Read the model definition and answer for the solid it produces. Units are mm, in the model's axes. Coordinates: 2 decimals unless noted, no trailing zeros. Loops run counter-clockwise (first coordinate to the right, second up) from the corner with the lowest first, then second, coordinate; pieces in that order, holes last. Notation, with made-up numbers: M 68,67.25 L 99,67.25 A22 cw 99,83.25 Z; hole C 41.5,55 d11. An arc over 180 degrees is marked long. Use one line per item in the form item = value. Start each with the question number.
1. Find the intervals of material crossed by probe 1 along Y at (x, z) = (0, 1.5); probe 2 along Z at (x, y) = (-20.5, 0); probe 3 along X at (y, z) = (6, 3), in increasing order. Write a range as [from, to].
2. The part is cut by section B-B (x = 80.5). Give the vertices of the cut face in (y, z), plus the area to 3 significant figures.
3. Flat-ended cylindrical pins translate along their axes: pin 1 (2.5 mm diameter, centred on x = -7.07, y = 7.07, fed in from +Z) (3 decimals); pin 2 (2 mm diameter, centred on x = 46, z = -2, fed in from +Y). Find the tip coordinate at first contact, or state that the pin passes through.
4. The part is cut by section A-A (z = 0). Give the number of separate pieces and of enclosed holes in the cut face, plus the area to 3 significant figures.
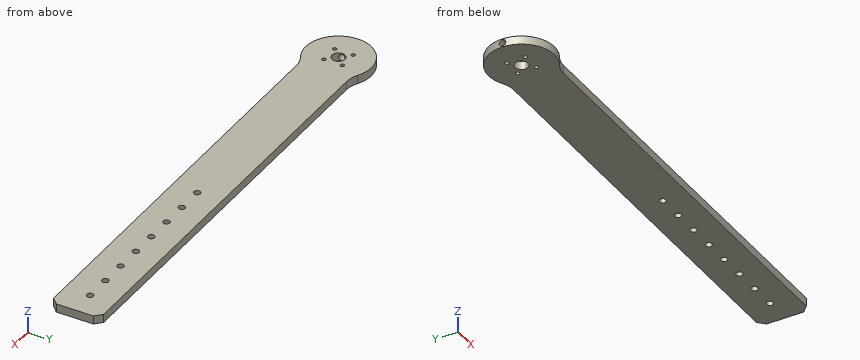
from build123d import *

# Parameters (mm, degrees)
SKETCH1_R           = 1.5
SKETCH1_R_2         = 2.5
SKETCH1_R_3         = 5
BOSS_EXTRUDE1_DEPTH = 3.2
SKETCH4_R           = 2.5
CUT_EXTRUDE1_DEPTH  = 32.4
FILLET1_R           = 20
CHAMFER1_SIZE       = 5


with BuildPart() as part:
    # Sketch1 → Boss-Extrude1 (new, symmetric)
    with BuildSketch(Plane.XY):
        with BuildLine():
            Line((345, 19.05), (16.189425561, 19.05))
            ThreePointArc((16.189425561, 19.05), (-25, 0), (16.189425561, -19.05))
            Line((16.189425561, -19.05), (345, -19.05))
            Line((345, -19.05), (345, 19.05))
        make_face()
        with Locations((7.071067812, 7.071067812)):
            Circle(SKETCH1_R, mode=Mode.SUBTRACT)
        with Locations((7.071067812, -7.071067812)):
            Circle(SKETCH1_R, mode=Mode.SUBTRACT)
        with Locations((-7.071067812, -7.071067812)):
            Circle(SKETCH1_R, mode=Mode.SUBTRACT)
        with Locations((-7.071067812, 7.071067812)):
            Circle(SKETCH1_R, mode=Mode.SUBTRACT)
        with Locations((325, 0)):
            Circle(SKETCH1_R_2, mode=Mode.SUBTRACT)
        with Locations((305, 0)):
            Circle(SKETCH1_R_2, mode=Mode.SUBTRACT)
        with Locations((285, 0)):
            Circle(SKETCH1_R_2, mode=Mode.SUBTRACT)
        with Locations((265, 0)):
            Circle(SKETCH1_R_2, mode=Mode.SUBTRACT)
        with Locations((245, 0)):
            Circle(SKETCH1_R_2, mode=Mode.SUBTRACT)
        with Locations((225, 0)):
            Circle(SKETCH1_R_2, mode=Mode.SUBTRACT)
        with Locations((205, 0)):
            Circle(SKETCH1_R_2, mode=Mode.SUBTRACT)
        with Locations((185, 0)):
            Circle(SKETCH1_R_2, mode=Mode.SUBTRACT)
        Circle(SKETCH1_R_3, mode=Mode.SUBTRACT)
    extrude(amount=BOSS_EXTRUDE1_DEPTH, both=True)

    # Sketch4 → Cut-Extrude1 (cut)
    with BuildSketch(Plane(origin=(0, 0, 0), x_dir=(0, 0, -1), z_dir=(1, 0, 0))):
        Circle(SKETCH4_R)
    extrude(amount=-CUT_EXTRUDE1_DEPTH, mode=Mode.SUBTRACT)

    # Fillet1
    fillet1_edges = [part.edges().sort_by_distance(p)[0] for p in [
        (16.189425561, -19.05, 0),
        (16.189425561, 19.05, 0),
    ]]
    fillet(fillet1_edges, radius=FILLET1_R)

    # Chamfer1
    chamfer1_edges = [part.edges().sort_by_distance(p)[0] for p in [
        (345, -19.05, 0),
        (345, 19.05, 0),
    ]]
    chamfer(chamfer1_edges, length=CHAMFER1_SIZE)


solid = part.part
Computed values:
q1.probe_1 = [-25, -5], [5, 25]
q1.probe_2 = [-3.2, -2.5], [2.5, 3.2]
q1.probe_3 = [-24.27, -8.12], [-6.02, 6.02], [8.12, 345]
q2.outline = M -19.05,-3.2 L 19.05,-3.2 L 19.05,3.2 L -19.05,3.2 Z
q2.area = 244 mm²
q3.pin_1 = through
q3.pin_2 = 19.05
q4.separate_pieces = 1
q4.enclosed_holes = 12
q4.area = 13,900 mm²
